Design review of the part built by this model. Coordinates are the model's own, in mm. A direction names the side the tool comes from. Give positions to 0.01 mm unless a question says otherwise; leave off trailing zeros. Order: outer loops, then holes, each group sorted by start corner. A loop starts at its lowest first (then second) coordinate and runs counter-clockwise, first axis right, second up. Notation, with made-up numbers: (87.5, 28.5) -> (104.5, 28.5) arc R27 ccw to (104.5, 44.5) -> close; hole circle Ø8 at (26, 89). An arc over 180 degrees is marked (long way). Return JSON: item names as keys, results as strings.
```python
from build123d import *

# Parameters (mm, degrees)
SKETCH1_W           = 56.05
SKETCH1_H           = 61.05
SKETCH1_W_2         = 50.05
SKETCH1_H_2         = 55.05
BOSS_EXTRUDE1_DEPTH = 3
SKETCH1_3_W         = 56.05
SKETCH1_3_H         = 61.05
SKETCH1_3_W_2       = 50.05
SKETCH1_3_H_2       = 55.05
BOSS_EXTRUDE2_DEPTH = 21
CUT_EXTRUDE1_REACH  = 58.05
SKETCH2_R           = 1.525
SKETCH2_W           = 6.5
SKETCH2_H           = 3.25
CUT_EXTRUDE2_REACH  = 63.05
SKETCH3_W           = 10.65
SKETCH3_H           = 7
SKETCH4_W           = 11.05
SKETCH4_H           = 7
CUT_EXTRUDE3_DEPTH  = 3
BOSS_EXTRUDE3_DEPTH = 4
FILLET1_R           = 2
SKETCH6_W           = 7.5
SKETCH6_H           = 4.25
CUT_EXTRUDE4_DEPTH  = 1.5


with BuildPart() as part:
    # Sketch1 → Boss-Extrude1 (new body)
    with BuildSketch(Plane(origin=(0, 0, 0), x_dir=(1, 0, 0), z_dir=(0, 1, 0))):
        Rectangle(SKETCH1_W, SKETCH1_H)
        Rectangle(SKETCH1_W_2, SKETCH1_H_2, mode=Mode.SUBTRACT)
        Rectangle(SKETCH1_W_2, SKETCH1_H_2)
    extrude(amount=BOSS_EXTRUDE1_DEPTH)

    # Sketch1_3 → Boss-Extrude2 (add)
    with BuildSketch(Plane(origin=(0, 0, 0), x_dir=(1, 0, 0), z_dir=(0, 1, 0))):
        Rectangle(SKETCH1_3_W, SKETCH1_3_H)
        Rectangle(SKETCH1_3_W_2, SKETCH1_3_H_2, mode=Mode.SUBTRACT)
    extrude(amount=BOSS_EXTRUDE2_DEPTH)

    # Sketch2 → Cut-Extrude1 (cut, up to next)
    with BuildSketch(Plane(origin=(28.025, 0, 0), x_dir=(0, 0, -1), z_dir=(1, 0, 0)), mode=Mode.PRIVATE) as cut_extrude1_sk1:
        with Locations((-24.025, 11.825)):
            Circle(SKETCH2_R)
    cut_extrude1_tool1 = extrude(cut_extrude1_sk1.sketch, amount=-CUT_EXTRUDE1_REACH, mode=Mode.PRIVATE) & part.part
    add(cut_extrude1_tool1.solids().sort_by_distance((28.025, 11.825, 24.025))[0], mode=Mode.SUBTRACT)
    # Sketch2 → Cut-Extrude1 (cut, up to next)
    with BuildSketch(Plane(origin=(28.025, 0, 0), x_dir=(0, 0, -1), z_dir=(1, 0, 0)), mode=Mode.PRIVATE) as cut_extrude1_sk2:
        with Locations((-9.975, 11.825)):
            Circle(SKETCH2_R)
    cut_extrude1_tool2 = extrude(cut_extrude1_sk2.sketch, amount=-CUT_EXTRUDE1_REACH, mode=Mode.PRIVATE) & part.part
    add(cut_extrude1_tool2.solids().sort_by_distance((28.025, 11.825, 9.975))[0], mode=Mode.SUBTRACT)
    # Sketch2 → Cut-Extrude1 (cut, up to next)
    with BuildSketch(Plane(origin=(28.025, 0, 0), x_dir=(0, 0, -1), z_dir=(1, 0, 0)), mode=Mode.PRIVATE) as cut_extrude1_sk3:
        with Locations((-17, 11.825)):
            Rectangle(SKETCH2_W, SKETCH2_H)
    cut_extrude1_tool3 = extrude(cut_extrude1_sk3.sketch, amount=-CUT_EXTRUDE1_REACH, mode=Mode.PRIVATE) & part.part
    add(cut_extrude1_tool3.solids().sort_by_distance((28.025, 11.825, 17))[0], mode=Mode.SUBTRACT)

    # Sketch3 → Cut-Extrude2 (cut, up to next)
    with BuildSketch(Plane(origin=(0, 0, -30.525), x_dir=(-1, 0, 0), z_dir=(0, 0, -1)), mode=Mode.PRIVATE) as cut_extrude2_sk1:
        with Locations((3.35, 13.5)):
            Rectangle(SKETCH3_W, SKETCH3_H)
    cut_extrude2_tool1 = extrude(cut_extrude2_sk1.sketch, amount=-CUT_EXTRUDE2_REACH, mode=Mode.PRIVATE) & part.part
    add(cut_extrude2_tool1.solids().sort_by_distance((-3.35, 13.5, -30.525))[0], mode=Mode.SUBTRACT)

    # Sketch4 → Cut-Extrude3 (cut)
    with BuildSketch(Plane.ZY.offset(28.025)):
        with Locations((18.54, 6)):
            Rectangle(SKETCH4_W, SKETCH4_H)
    extrude(amount=-CUT_EXTRUDE3_DEPTH, mode=Mode.SUBTRACT)

    # Sketch5 → Boss-Extrude3 (add)
    with BuildSketch(Plane(origin=(0, 3, 0), x_dir=(1, 0, 0), z_dir=(0, 1, 0))):
        Polygon((5.475, -7.615), (-25.025, -7.615), (-25.025, -10.115), (2.975, -10.115), (2.975, -27.525), (5.475, -27.525), align=None)
    extrude(amount=BOSS_EXTRUDE3_DEPTH)

    # Fillet1
    fillet1_edges = [part.edges().sort_by_distance(p)[0] for p in [
        (-28.025, 0, 0),
        (0, 0, -30.525),
        (28.025, 0, 0),
        (0, 0, 30.525),
        (-28.025, 10.5, 30.525),
        (-28.025, 10.5, -30.525),
        (28.025, 10.5, -30.525),
        (28.025, 10.5, 30.525),
    ]]
    fillet(fillet1_edges, radius=FILLET1_R)

    # Sketch6 → Cut-Extrude4 (cut)
    with BuildSketch(Plane(origin=(28.025, 0, 0), x_dir=(0, 0, -1), z_dir=(1, 0, 0))):
        with Locations((-17, 11.825)):
            Rectangle(SKETCH6_W, SKETCH6_H)
    extrude(amount=-CUT_EXTRUDE4_DEPTH, mode=Mode.SUBTRACT)


solid = part.part
```
Item 1: Add section B-B (z = 16). Give the boundary of the cut face in (x, y) (3 decimals).
Result set:
{"outline": "(-28.025, 2) arc R2 ccw to (-26.025, 0) -> (26.025, 0) arc R2 ccw to (28.025, 2) -> (28.025, 9.7) -> (26.525, 9.7) -> (26.525, 10.2) -> (25.025, 10.2) -> (25.025, 3) -> (5.475, 3) -> (5.475, 7) -> (2.975, 7) -> (2.975, 3) -> (-25.025, 3) -> (-25.025, 2.5) -> (-28.025, 2.5) -> close; (-28.025, 9.5) -> (-25.025, 9.5) -> (-25.025, 21) -> (-28.025, 21) -> close; (25.025, 13.45) -> (26.525, 13.45) -> (26.525, 13.95) -> (28.025, 13.95) -> (28.025, 21) -> (25.025, 21) -> close"}
Item 2: Add section D-D (x = 4.5). Give the boundary of the cut face in (y, z) (3 decimals), plus the area to 3 significant figures.
Result set:
{"outline": "(0, -28.525) arc R2 ccw to (2, -30.525) -> (21, -30.525) -> (21, -27.525) -> (3, -27.525) -> (3, 7.615) -> (7, 7.615) -> (7, 27.525) -> (21, 27.525) -> (21, 30.525) -> (2, 30.525) arc R2 ccw to (0, 28.525) -> close", "area": "369 mm^2"}
Item 3: Add section A-A (x = -6). Give the boundary of the cut face in (y, z) (3 decimals).
Result set:
{"outline": "(0, -28.525) arc R2 ccw to (2, -30.525) -> (10, -30.525) -> (10, -27.525) -> (3, -27.525) -> (3, 7.615) -> (7, 7.615) -> (7, 10.115) -> (3, 10.115) -> (3, 27.525) -> (21, 27.525) -> (21, 30.525) -> (2, 30.525) arc R2 ccw to (0, 28.525) -> close; (17, -30.525) -> (21, -30.525) -> (21, -27.525) -> (17, -27.525) -> close"}
Item 4: Add section C-C (y = 15). Give the boundary of the cut face in (x, z) (3 decimals), plus the area to 3 significant figures.
Result set:
{"outline": "(-28.025, -28.525) arc R2 ccw to (-26.025, -30.525) -> (-8.675, -30.525) -> (-8.675, -27.525) -> (-25.025, -27.525) -> (-25.025, 27.525) -> (25.025, 27.525) -> (25.025, -27.525) -> (1.975, -27.525) -> (1.975, -30.525) -> (26.025, -30.525) arc R2 ccw to (28.025, -28.525) -> (28.025, 28.525) arc R2 ccw to (26.025, 30.525) -> (-26.025, 30.525) arc R2 ccw to (-28.025, 28.525) -> close", "area": "631 mm^2"}
Item 5: Machinability: for faces 1 (the face through (28.025, 11, 0)), 2 (the face through (-27, 6, 13.015)), 3 (the face through (2.975, 5, 19)), 4 (the face through (27, 12, 13.25)), which of the approach directions +Z, -Z, +X, -X, +Y, -Y give a long, thin tool a straight path to every point of the face, cutting with its end or side? Answer none if there is none.
Result set:
{"face 1": "+Z, -Z, +X, +Y, -Y", "face 2": "-X", "face 3": "+Y", "face 4": "+X"}
Item 6: For pin 1 (10 mm diameter, centred on x = -13, z = 12.5, fed in from +Y); pin 2 (1.5 mm diameter, centred on y = 14.5, z = -29.5, fed in from -X); pin 3 (8 mm diameter, centred on x = -6.5, z = -19.5, fed in from +Y), all flat-tipped, find the tip position at first contact; note any pin that passes through.
Result set:
{"pin 1": "stops at y = 7", "pin 2": "stops at x = -28.01", "pin 3": "stops at y = 3"}
Item 7: Wall thickness on L1, parallel to X at y = 8, z = -7.5 (3 decimals); L2, parallel to Z at x = -24.5, y = 6.5 (3 decimals); L3, parallel to Z at x = -17, y = 17.5 (3 decimals): over which ranges is each line inside the solid? List them lowest first. Write a range as [from, to].
Result set:
{"L1": "x = [-28.025, -25.025], [25.025, 28.025]", "L2": "z = [-30.525, -27.525], [7.615, 10.115], [27.525, 30.525]", "L3": "z = [-30.525, -27.525], [27.525, 30.525]"}
Item 8: Mouldability with a two-part tool opening along X and no side actions: class faces 5 (the face through (-27.455, 11.633, 29.924)), 6 (the face through (1.975, 13, -29)), 7 (the face through (27.424, 11.367, -29.955)) as released by +X, released by -X, zero draft, split by the parting line, or undercut.
Result set:
{"face 5": "released by -X", "face 6": "undercut", "face 7": "released by +X"}
